Check sheet for the modelled part. Datum: model origin and axes. Units: mm. A direction names the side the tool comes from. Round coordinates to 2 decimals unless told otherwise and drop trailing zeros. Write each loop counter-clockwise with the first axis right and the second up, starting at its lowest first coordinate (ties: lowest second). Pieces come first, ordered by that corner, then holes. Notation, with made-up numbers: (15.5, 11.25) - (57.5, 11.25) arc R30 ccw to (57.5, 34.25) - close; hole circle Ø6 at (16, 86.5). An arc over 180 degrees is marked (long way). Answer as a JSON object with one key per item and string values. Group by question number.
Item 1: Sectioned sample at C-C on y = 5.5. Count the separate pieces of the cut face and the enclosed holes in it, plus the area to 3 significant figures.
Item 2: Sectioned sample at D-D on x = 16.5. Record the boundary of the cut face in (y, z).
Item 3: Release check for a two-part mould opening along X. For faces 4 (the cylindrical face through (24.1, 5.07, -5.14)), 5 (the cylindrical face through (40.5, 5.1, 0.1)), 6 (the flat face through (-1, 0, 11)) record: pulls with the +X half, pulls with the -X half, needs draft (parallel to the pull), parting line crosses it, or undercut.
Item 4: Set-up check for faces 1 (the flat face through (0, 5, 6)), 2 (the cylindrical face through (-25.522, 8.311, -22.579)), 3 (the flat face through (-1, 10, 11)): record each of +Z, -Z, +X, -X, +Y, -Y from which the full face is reachable in a straight line by a thin tool's end or side.
Item 5: Thickness scan on line 1 (X direction, y = 5, z = 20); line 2 (Z direction, x = -27.5, y = 5); line 3 (X direction, y = 3, z = 12.5) (3 decimals). Record the ranges inside material, lowest first.
Item 6: Gauge pin test, flat ends, axial feed: P1, Ø1.5, axis at y = 8.5, z = -6.5, coming from the -X side; P2, Ø2.5, axis at x = -27.5, z = 20, coming from the -Y side; P3, Ø3, axis at y = 4, z = 13.5, coming from the +X side; P4, Ø2.5, axis at x = 32.5, z = 0, coming from the +Y side. Record the tip position at first contact, or that the pin passes through.
Item 7: Sectioned sample at B-B on z = 13. Record the boundary of the cut face in (x, y).
Item 8: Sectioned sample at A-A on x = 27.5. Record the boundary of the cut face in (y, z) (3 decimals), plus the area to 3 significant figures.
```python
from build123d import *

# Parameters (mm, degrees)
SKETCH1_W                                    = 65
SKETCH1_H                                    = 50
SKETCH1_R                                    = 3.05
BOSS_EXTRUDE1_DEPTH                          = 10
FILLET1_R                                    = 3
CBORE_FOR_M3_HEX_SOCKET_HEAD_CAP_SCR_2_COUNT = 2
CBORE_FOR_M3_HEX_SOCKET_HEAD_CAP_SCR_2_PITCH = 55
CBORE_FOR_M3_HEX_SOCKET_HEAD_CAP_SCR_3_COUNT = 2
CBORE_FOR_M3_HEX_SOCKET_HEAD_CAP_SCR_3_PITCH = 68.007352544
CBORE_FOR_M3_HEX_SOCKET_HEAD_CAP_SCR_4_COUNT = 2
CBORE_FOR_M3_HEX_SOCKET_HEAD_CAP_SCR_4_PITCH = 40
SKETCH6_R                                    = 8
BOSS_EXTRUDE2_DEPTH                          = 10
FILLET2_R                                    = 3
F_2_9_2_9_DIAMETER_HOLE1_D                   = 2.9
F_2_9_2_9_DIAMETER_HOLE1_DEPTH               = 6
F_2_9_2_9_DIAMETER_HOLE1_CSINK_D             = 2.95
F_2_9_2_9_DIAMETER_HOLE1_CSINK_ANGLE         = 90
F_2_9_2_9_DIAMETER_HOLE1_TIP                 = 0.871247898
CUT_EXTRUDE1_DEPTH                           = 10


with BuildPart() as part:
    # Sketch1 → Boss-Extrude1 (new body)
    with BuildSketch(Plane(origin=(0, 0, 0), x_dir=(1, 0, 0), z_dir=(0, 1, 0))):
        Rectangle(SKETCH1_W, SKETCH1_H)
        with Locations(Location((-12.375, 12.5, 0), (0, 0, 270))):
            Circle(SKETCH1_R, mode=Mode.SUBTRACT)
        with Locations(Location((-12.375, -12.5, 0), (0, 0, 270))):
            Circle(SKETCH1_R, mode=Mode.SUBTRACT)
        with Locations(Location((12.375, 12.5, 0), (0, 0, 270))):
            Circle(SKETCH1_R, mode=Mode.SUBTRACT)
        with Locations(Location((12.375, -12.5, 0), (0, 0, 270))):
            Circle(SKETCH1_R, mode=Mode.SUBTRACT)
    extrude(amount=BOSS_EXTRUDE1_DEPTH)

    # Fillet1
    fillet1_edges = [part.edges().sort_by_distance(p)[0] for p in [
        (32.5, 5, 25),
        (-32.5, 5, 25),
        (-32.5, 5, -25),
        (32.5, 5, -25),
    ]]
    fillet(fillet1_edges, radius=FILLET1_R)

    # Sketch3 → CBORE for M3 Hex Socket Head Cap Screw1 (revolve, cut)
    with BuildSketch(Plane(origin=(27.5, 10, -20), x_dir=(0, 0, 1), z_dir=(1, 0, 0))):
        Polygon((0, 0), (0, 10), (1.7, 10), (1.7, 3.4), (3.25, 3.4), (3.25, 0.025), (3.275, 0), align=None)
    cbore_for_m3_hex_socket_head_cap_screw1 = revolve(axis=Axis((27.5, 16.35, -20), (0, -1, 0)), mode=Mode.SUBTRACT)

    # CBORE for M3 Hex Socket Head Cap Scr 2: CBORE for M3 Hex Socket Head Cap Screw1 ×2
    with Locations(*[(-i * CBORE_FOR_M3_HEX_SOCKET_HEAD_CAP_SCR_2_PITCH, 0, 0) for i in range(1, CBORE_FOR_M3_HEX_SOCKET_HEAD_CAP_SCR_2_COUNT)]):
        add(cbore_for_m3_hex_socket_head_cap_screw1, mode=Mode.SUBTRACT)

    # CBORE for M3 Hex Socket Head Cap Scr 3: CBORE for M3 Hex Socket Head Cap Screw1 ×2
    with Locations(*[Vector(-0.8087360843031886, 0, 0.5881716976750463) * (i * CBORE_FOR_M3_HEX_SOCKET_HEAD_CAP_SCR_3_PITCH) for i in range(1, CBORE_FOR_M3_HEX_SOCKET_HEAD_CAP_SCR_3_COUNT)]):
        add(cbore_for_m3_hex_socket_head_cap_screw1, mode=Mode.SUBTRACT)

    # CBORE for M3 Hex Socket Head Cap Scr 4: CBORE for M3 Hex Socket Head Cap Screw1 ×2
    with Locations(*[(0, 0, i * CBORE_FOR_M3_HEX_SOCKET_HEAD_CAP_SCR_4_PITCH) for i in range(1, CBORE_FOR_M3_HEX_SOCKET_HEAD_CAP_SCR_4_COUNT)]):
        add(cbore_for_m3_hex_socket_head_cap_screw1, mode=Mode.SUBTRACT)

    # Sketch6 → Boss-Extrude2 (add)
    with BuildSketch(Plane(origin=(0, 10, 0), x_dir=(1, 0, 0), z_dir=(0, 1, 0))):
        with Locations((-32.5, 0)):
            Circle(SKETCH6_R)
        with Locations((32.5, 0)):
            Circle(SKETCH6_R)
    extrude(amount=-BOSS_EXTRUDE2_DEPTH)

    # Fillet2
    fillet2_edges = [part.edges().sort_by_distance(p)[0] for p in [
        (32.5, 5, -8),
        (32.5, 5, 8),
        (-32.5, 5, 8),
        (-32.5, 5, -8),
    ]]
    fillet(fillet2_edges, radius=FILLET2_R)

    # Ø2.9 (2.9) Diameter Hole1
    with Locations(Plane(origin=(0, 10, 0), x_dir=(1, 0, 0), z_dir=(0, 1, 0))):
        with Locations((-32.5, 0), (32.5, 0)):
            CounterSinkHole(F_2_9_2_9_DIAMETER_HOLE1_D / 2, F_2_9_2_9_DIAMETER_HOLE1_CSINK_D / 2, depth=F_2_9_2_9_DIAMETER_HOLE1_DEPTH, counter_sink_angle=F_2_9_2_9_DIAMETER_HOLE1_CSINK_ANGLE)
            with Locations((0, 0, -(F_2_9_2_9_DIAMETER_HOLE1_DEPTH + F_2_9_2_9_DIAMETER_HOLE1_TIP / 2))):  # 118° drill point
                Cone(0, F_2_9_2_9_DIAMETER_HOLE1_D / 2, F_2_9_2_9_DIAMETER_HOLE1_TIP, mode=Mode.SUBTRACT)

    # Sketch9 → Cut-Extrude1 (cut)
    with BuildSketch(Plane(origin=(0, 10, 0), x_dir=(1, 0, 0), z_dir=(0, 1, 0))):
        with BuildLine():
            Line((-22, 6), (22, 6))
            ThreePointArc((22, 6), (24.121320344, 5.121320344), (25, 3))
            Line((25, 3), (25, -3))
            ThreePointArc((25, -3), (24.121320344, -5.121320344), (22, -6))
            Line((22, -6), (-22, -6))
            ThreePointArc((-22, -6), (-24.121320344, -5.121320344), (-25, -3))
            Line((-25, -3), (-25, 3))
            ThreePointArc((-25, 3), (-24.121320344, 5.121320344), (-22, 6))
        make_face()
    extrude(amount=-CUT_EXTRUDE1_DEPTH, mode=Mode.SUBTRACT)


solid = part.part
```
Completed:
{
 "1": {"separate pieces": "1", "enclosed holes": "11", "area": "2,690 mm²"},
 "2": {"outline": "(0, -25) - (10, -25) - (10, -6) - (0, -6) - close; (0, 6) - (10, 6) - (10, 25) - (0, 25) - close"},
 "3": {"face 4": "undercut", "face 5": "pulls with the +X half", "face 6": "needs draft"},
 "4": {"face 1": "+Y, -Y", "face 2": "+Y", "face 3": "+Z, -Z, +X, -X, +Y"},
 "5": {"line 1": "-32.5 to -29.2, -25.8 to 25.8, 29.2 to 32.5", "line 2": "-25 to -21.7, -18.3 to 18.3, 21.7 to 25", "line 3": "-32.5 to -15.425, -9.325 to 9.325, 15.425 to 32.5"},
 "6": {"P1": "x = -38.06", "P2": "through", "P3": "x = 32.5", "P4": "y = 3.88"},
 "7": {"outline": "(-32.5, 0) - (-15.38, 0) - (-15.38, 10) - (-32.5, 10) - close; (-9.37, 0) - (9.37, 0) - (9.37, 10) - (-9.37, 10) - close; (15.38, 0) - (32.5, 0) - (32.5, 10) - (15.38, 10) - close"},
 "8": {"outline": "(0, -25) - (10, -25) - (10, -23.275) - (9.975, -23.25) - (6.6, -23.25) - (6.6, -21.7) - (0, -21.7) - close; (0, -18.3) - (6.6, -18.3) - (6.6, -16.75) - (9.975, -16.75) - (10, -16.725) - (10, 16.725) - (9.975, 16.75) - (6.6, 16.75) - (6.6, 18.3) - (0, 18.3) - close; (0, 21.7) - (6.6, 21.7) - (6.6, 23.25) - (9.975, 23.25) - (10, 23.275) - (10, 25) - (0, 25) - close", "area": "411 mm²"}
}
